```python
from build123d import *

# Parameters (mm, degrees)
F1_DEPTH = 12.7
F2_T     = -2.54
F3_W     = 9.652
F3_H     = 4.445
F4_DEPTH = 25.4


with BuildPart() as f1:
    # F0 (on Front) → F1 (new body)
    with BuildSketch(Plane.XZ):
        Polygon((-47.413333, 38.1), (-47.413333, 0), (41.486667, 0), (41.486667, 38.1), (22.436667, 21.299479), (-28.363333, 21.299479), align=None)
    extrude(amount=-F1_DEPTH)

    # F2
    f2_openings = [f1.faces().sort_by_distance(p)[0] for p in [
        (-2.963333, 6.35, 21.299479),
        (-37.888333, 6.35, 29.69974),
        (31.961667, 6.35, 29.69974),
    ]]
    offset(amount=F2_T, openings=f2_openings)

    # F3 (on Top) → F4 (cut)
    with BuildSketch(Plane.XY):
        with Locations((-2.963333, 6.866706)):
            Rectangle(F3_W, F3_H)
    extrude(amount=F4_DEPTH, mode=Mode.SUBTRACT)


solid = f1.part
```
Can you work these out from the model? Positions are in its coordinate system, mm. A direction names the side the tool comes from. Round coordinates to 2 decimals unless told otherwise and drop trailing zeros. Order: outer loops, then holes, each group sorted by start corner. A loop starts at its lowest first (then second) coordinate and runs counter-clockwise, first axis right, second up.
(1) If we section it at B-B (z = 16.5): Please give me the cut outline in (x, y), plus the area to 3 significant figures.
Results are:
outline: (-47.41, 0) - (41.49, 0) - (41.49, 12.7) - (-47.41, 12.7) - close; hole (-44.87, 2.54) - (38.95, 2.54) - (38.95, 10.16) - (-44.87, 10.16) - close
area: 490 mm2
(2) If we section it at D-D (x = -10): Please give me the cut outline in (y, z).
Results are:
outline: (0, 0) - (12.7, 0) - (12.7, 21.3) - (10.16, 21.3) - (10.16, 2.54) - (2.54, 2.54) - (2.54, 21.3) - (0, 21.3) - close
(3) If we section it at A-A (x = -1): Please give me the cut outline in (y, z), plus the area to 3 significant figures.
Results are:
outline: (0, 0) - (4.64, 0) - (4.64, 2.54) - (2.54, 2.54) - (2.54, 21.3) - (0, 21.3) - close; (9.09, 0) - (12.7, 0) - (12.7, 21.3) - (10.16, 21.3) - (10.16, 2.54) - (9.09, 2.54) - close
area: 116 mm2
(4) If I drill on L1, parallel to X at y = 5.25, z = 34; L2, parallel to Y at x = -32, z = 23; L3, parallel to X at y = 5, z = 2, over which ranges is the centre line in solid material (lowest first)?
Results are:
L1: x = -47.41 to -44.87, 38.95 to 41.49
L2: y = 0 to 2.54, 10.16 to 12.7
L3: x = -47.41 to -7.79, 1.86 to 41.49
(5) If we section it at C-C (y = 7.5): Please give me the cut outline in (x, z), plus the area to 3 significant figures.
Results are:
outline: (-47.41, 0) - (-7.79, 0) - (-7.79, 2.54) - (-44.87, 2.54) - (-44.87, 35.86) - (-47.41, 38.1) - close; (1.86, 0) - (41.49, 0) - (41.49, 38.1) - (38.95, 35.86) - (38.95, 2.54) - (1.86, 2.54) - close
area: 376 mm2
(6) We'd pull the mould along X, two halves only. Please class faces 5 (the face through (-4, 12.7, 15)), 6 (the face through (-3, 4.644, 1)), 7 (the face through (-47.413, 6, 19)): +X half, -X half, draft (parallel to the pull), parting line (faces both ways), or undercut.
Results are:
face 5: draft
face 6: undercut
face 7: -X half
(7) On a 3-axis mill with a long thin cutter (end or side, diameter ignored), from which of +Z, -Z, +X, -X, +Y, -Y can I reach the whole of each face in a straight line? I mean faces 1 (the face through (-7.789, 7, 1)), 2 (the face through (-4, 3, 0)), 3 (the face through (-4, 4, 2.54)), 4 (the face through (32.1, 2.03, 29.82)). Say none if no direction works.
Results are:
face 1: +Z, -Z
face 2: -Z, +X, -X, +Y, -Y
face 3: +Z
face 4: +Z, +Y, -Y
(8) I'm going to push flat-ended pins straight in: pin 1 (2 mm diameter, centred on x = -4.5, y = 11.5, fed in from +Z); pin 2 (2.5 mm diameter, centred on x = -10, y = 6, fed in from +Z); pin 3 (1 mm diameter, centred on x = -23, z = 22, fed in from -Y). Where does each tip first touch, or does it pass through?
Results are:
pin 1: stops at z = 21.3
pin 2: stops at z = 2.54
pin 3: passes through
